Check sheet for the drawn part. Datum: minimum x, y, z corner. Units: mm. A direction names the side the tool comes from. Round coordinates to 2 decimals unless told otherwise and drop trailing zeros. Loops run counter-clockwise (first coordinate to the right, second up) from the corner with the lowest first, then second, coordinate; pieces in that order, holes last.
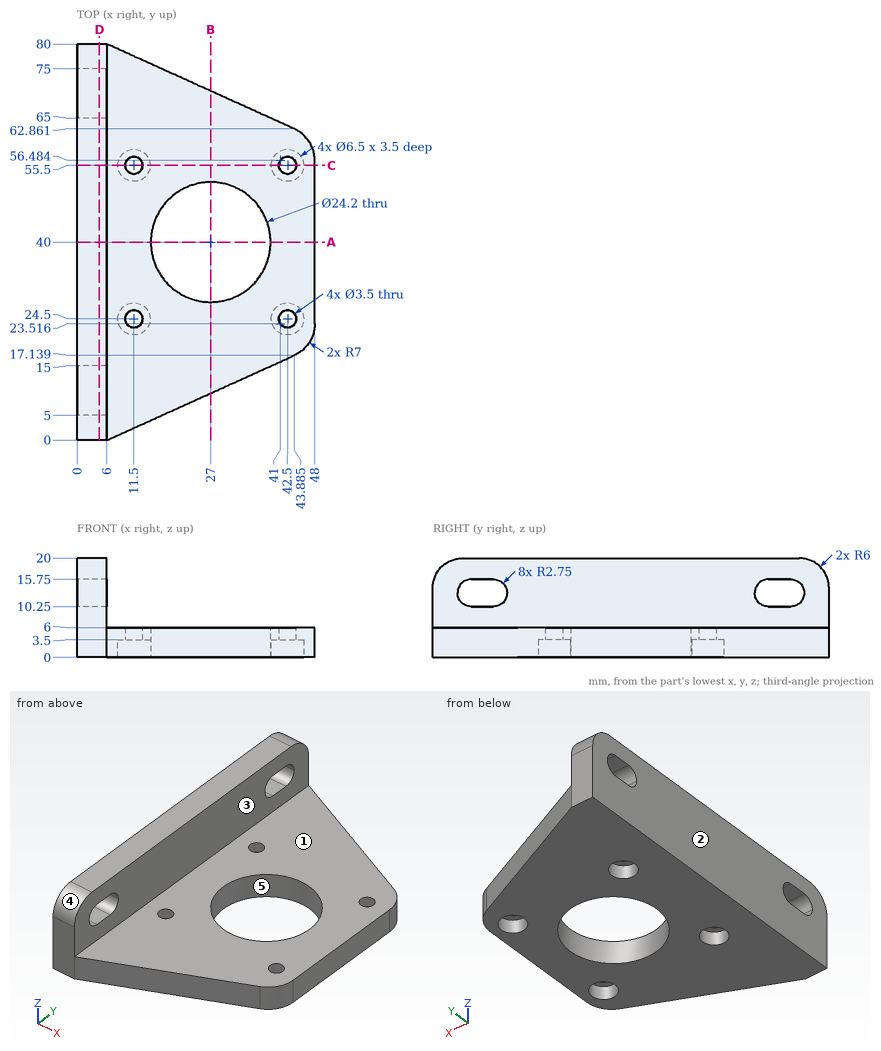
1) Sectioned sample at A-A, the plane y = 40. Record the cut outline in (x, z), then the cut area to 3 significant figures.
Report:
outline: (0, 0) - (14.9, 0) - (14.9, 6) - (6, 6) - (6, 20) - (0, 20) - close; (39.1, 0) - (48, 0) - (48, 6) - (39.1, 6) - close
area: 227 mm2
2) Access from +Z, -Z, +X, -X, +Y, -Y to the whole of each face (thin tool, end or side, straight path). Record for the marked faces 1 and 2.
Report:
face 1: +Z, +X, +Y, -Y
face 2: +Z, -Z, -X, +Y, -Y
3) Sectioned sample at C-C, the plane y = 55.5. Record the cut outline in (x, z).
Report:
outline: (0, 0) - (8.25, 0) - (8.25, 3.5) - (9.75, 3.5) - (9.75, 6) - (6, 6) - (6, 20) - (0, 20) - close; (13.25, 3.5) - (14.75, 3.5) - (14.75, 0) - (39.25, 0) - (39.25, 3.5) - (40.75, 3.5) - (40.75, 6) - (13.25, 6) - close; (44.25, 3.5) - (45.75, 3.5) - (45.75, 0) - (48, 0) - (48, 6) - (44.25, 6) - close
4) Gauge pin test, flat ends, axial feed: pin 1 (4 mm diameter, centred on y = 17.5, z = 10.5, fed in from +X); pin 2 (6 mm diameter, centred on x = 11.5, y = 24.5, fed in from -Z); pin 3 (10.5 mm diameter, centred on x = 42.5, y = 24.5, fed in from +Z). Record the tip position at first contact, or that the pin passes through.
Report:
pin 1: stops at x = 6
pin 2: stops at z = 3.5
pin 3: stops at z = 6
5) Mould release check, pull along Y, two halves, no side actions. Record for the marked faces 3, 4 and 5: +Y half, -Y half, draft (parallel to the pull), parting line (faces both ways), or undercut.
Report:
face 3: draft
face 4: -Y half
face 5: undercut
6) Sectioned sample at D-D, the plane x = 4.5. State how many separate pieces and enclosed holes the cut face has, then the cut area to 3 significant figures.
Report:
separate pieces: 1
enclosed holes: 2
area: 1,490 mm2
7) Scan lines: line 1 along X through (y, z) = (24.5, 4.5); line 2 along Y through (x, z) = (11.5, 2.45); line 3 along X through (y, z) = (26.5, 1.25). Record each from-to range of solid material in increasing order.
Report:
line 1: x = 0 to 9.75, 13.25 to 40.75, 44.25 to 48
line 2: y = 2.49 to 21.25, 27.75 to 52.25, 58.75 to 77.51
line 3: x = 0 to 8.94, 14.06 to 39.94, 45.06 to 48
8) Sectioned sample at B-B, the plane x = 27. Record the cut outline in (y, z), then the cut area to 3 significant figures.
Report:
outline: (9.5, 0) - (27.9, 0) - (27.9, 6) - (9.5, 6) - close; (52.1, 0) - (70.5, 0) - (70.5, 6) - (52.1, 6) - close
area: 221 mm2
